Could you check a few things on this drawing? It's one solid part, dimensions in mm from its lowest x, y, z. Round coordinates to 2 decimals unless told otherwise and drop trailing zeros. Loops run counter-clockwise (first coordinate to the right, second up) from the corner with the lowest first, then second, coordinate; pieces in that order, holes last. Notation, with made-up numbers: (-28.75, -13) -> (-3.75, -13) arc R25 cw to (-3.75, 24) -> close; hole circle Ø7 at (84.5, 7). An arc over 180 degrees is marked (long way). Put each result on its own line as item: value. Start each with the question number.
1. Imagine slicing it at A-A, the plane z = 165. Please give me the cut outline in (x, y).
2. I'm going to push flat-ended pins straight in: P1, Ø3, axis at x = 187, y = 3.5, coming from the -Z side; P2, Ø2, axis at y = 3, z = 236, coming from the +X side (1 decimal); P3, Ø1.5, axis at y = 2, z = 211, coming from the -X side. Where does each tip first touch, or does it pass through?
3. Imagine slicing it at C-C, the plane x = 273. Please give me the cut outline in (y, z).
4. Imagine slicing it at B-B, the plane y = 1.75. Please give me the cut outline in (x, z), and give its area (3 significant figures).
5. I need wall thicknesses on line 1 (X direction, y = 3.5, z = 165); line 2 (X direction, y = 6, z = 188.5) (1 decimal). Which ranges of each line are inside material? Lowest first, please. Write a range as [from, to].
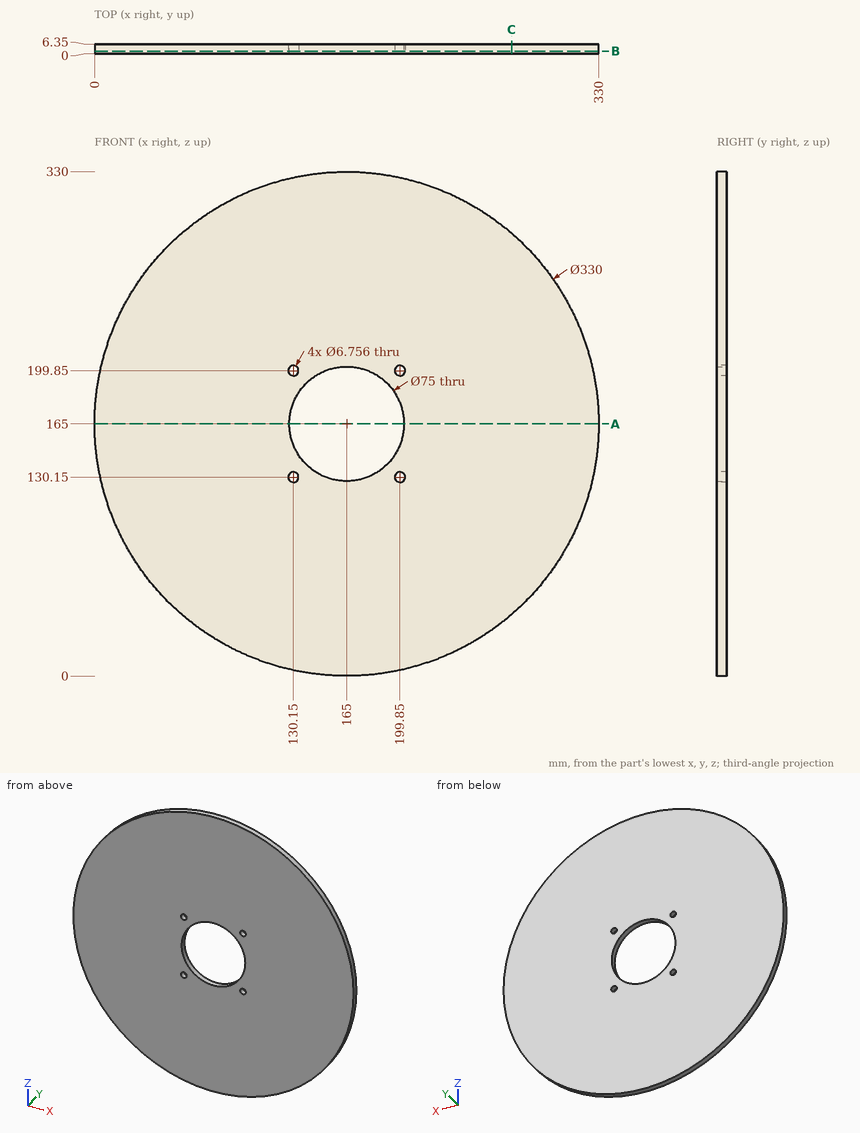
Entries:
1. outline: (0, 0) -> (127.5, 0) -> (127.5, 6.35) -> (0, 6.35) -> close; (202.5, 0) -> (330, 0) -> (330, 6.35) -> (202.5, 6.35) -> close
2. P1: z = 1.28
2. P2: x = 314.4
2. P3: x = 6.33
3. outline: (0, 40.26) -> (6.35, 40.26) -> (6.35, 289.74) -> (0, 289.74) -> close
4. outline: circle Ø330 at (165, 165); hole circle Ø6.76 at (130.15, 130.15); hole circle Ø6.76 at (130.15, 199.85); hole circle Ø75 at (165, 165); hole circle Ø6.76 at (199.85, 130.15); hole circle Ø6.76 at (199.85, 199.85)
4. area: 81,000 mm^2
5. line 1: [0, 127.5], [202.5, 330]
5. line 2: [1.7, 135.8], [194.2, 328.3]
